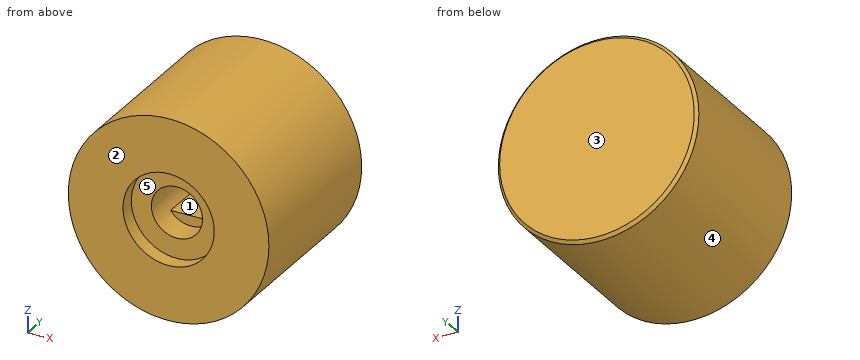
Autodesk Fusion 360 part; units mm, degrees
sketch "Sketch1" plane through (0, 0, 0) normal (0, 1, 0) x (1, 0, 0)
  circle A0 centre (0, 0) radius 10
  circle A1 centre (0, 0) radius 4.55
  circle A2 centre (0, 0) radius 2.545
  line L0 (0, 1.52) -> (2.0412, 1.52)
  line L1 (0, 1.52) -> (-2.0412, 1.52)
  line L2 (0, -1.52) -> (-2.0412, -1.52)
  line L3 (0, -1.52) -> (2.0412, -1.52)
  dimension "d1" = 20
  dimension "d2" = 9.1
  dimension "d3" = 5.09
  dimension "d4" = 1.52
  dimension "d6" = 1.52
extrude "Extrude1" add sketch "Sketch1" along normal blind 17 contours A0 | A1 | A2 L0 L1 L2 L3 | A2 L0 L1 | A2 L2 L3
extrude "Extrude2" cut sketch "Sketch1" along normal blind 10 contours A2 L0 L1 L2 L3
extrude "Extrude3" cut sketch "Sketch1" along normal blind 4.05 contours A2 L0 L1 | A2 L2 L3
extrude "Extrude4" cut sketch "Sketch1" along normal blind 1.5 contours A1
chamfer "Chamfer1" distance 0.3 angle 45 1 edges at (-9.3233, 17, 3.6162)
Can you work these out from the model? Positions are in its coordinate system, mm. Face numbers are marked on the shaded views. A direction names the side the tool comes from. Coordinates: 2 decimals unless noted, no trailing zeros. Order: outer loops, then holes, each group sorted by start corner. A loop starts at its lowest first (then second) coordinate and runs counter-clockwise, first axis right, second up. Notation, with made-up numbers: (52, -33) - (79, -33) arc R8 ccw to (79, -29) - close; hole circle Ø5 at (68.25, -36.5). An arc over 180 degrees is marked (long way). Answer as a JSON object with one key per item and string values. Group by question number.
Q1. We'd pull the mould along X, two halves only. Please class the marked faces 3, 4 and 5: +X half, -X half, draft (parallel to the pull), parting line (faces both ways), or undercut.
Q2. Will these pins go through, and if not, where does the flat tip stop? P1, Ø0.8, axis at x = 0.5, z = -2, coming from the -Y side; P2, Ø6, axis at y = 3.5, z = -6.5, coming from the -X side; P3, Ø2, axis at y = 8, z = 2, coming from the +X side.
Q3. Imagine slicing it at B-B (z = 0). Please give me the cut outline in (x, y) (3 decimals), and give its area (3 significant figures).
Q4. I need wall thicknesses on line 1 (X direction, y = 8, z = 0) (3 decimals); line 2 (X direction, y = 0.9, z = 0). Which ranges of each line are inside material? Lowest first, please. Write a range as from..to.
Q5. Imagine slicing it at A-A (x = 0). Please give me the cut outline in (y, z) (3 decimals).
Q6. Imagine slicing it at D-D (y = 12.5). Please give me the cut outline in (x, z).
Q7. On a 3-axis mill with a long thin cutter (end or side, diameter ignored), from which of +Z, -Z, +X, -X, +Y, -Y can I reach the whole of each face in a straight line? I mean the marked faces 1 and 2. Say none if no direction works.
Q8. Imagine slicing it at C-C (y = 2). Please give me the cut outline in (x, z) (3 decimals).
Determined:
{
 "1": {"face 3": "draft", "face 4": "parting line", "face 5": "undercut"},
 "2": {"P1": "stops at y = 4.05", "P2": "stops at x = -9.37", "P3": "stops at x = 9.95"},
 "3": {"outline": "(-10, 0) - (-4.55, 0) - (-4.55, 1.5) - (-2.545, 1.5) - (-2.545, 10) - (2.545, 10) - (2.545, 1.5) - (4.55, 1.5) - (4.55, 0) - (10, 0) - (10, 16.7) - (9.7, 17) - (-9.7, 17) - (-10, 16.7) - close", "area": "283 mm2"},
 "4": {"line 1": "x = -10..-2.545, 2.545..10", "line 2": "x = -10..-4.55, 4.55..10"},
 "5": {"outline": "(0, -10) - (16.7, -10) - (17, -9.7) - (17, 9.7) - (16.7, 10) - (0, 10) - (0, 4.55) - (1.5, 4.55) - (1.5, 2.545) - (4.05, 2.545) - (4.05, 1.52) - (10, 1.52) - (10, -1.52) - (4.05, -1.52) - (4.05, -2.545) - (1.5, -2.545) - (1.5, -4.55) - (0, -4.55) - close"},
 "6": {"outline": "circle Ø20 at (0, 0)"},
 "7": {"face 1": "-Y", "face 2": "+Z, -Z, +X, -X, -Y"},
 "8": {"outline": "circle Ø20 at (0, 0); hole circle Ø5.09 at (0, 0)"}
}
